The figure shows three views and two pictorial views of one solid part (mm, origin at its lowest corner). Answer the questions. A direction names the side the tool comes from. Coordinates: 2 decimals unless noted, no trailing zeros. Write each loop counter-clockwise with the first axis right and the second up, starting at its lowest first coordinate (ties: lowest second). Pieces come first, ordered by that corner, then holes. Notation, with made-up numbers: M 32.5,53.5 L 47.5,53.5 A14 cw 47.5,80.5 Z; hole C -14.5,58.25 d8. An arc over 180 degrees is marked long. Write item = value, one per line.
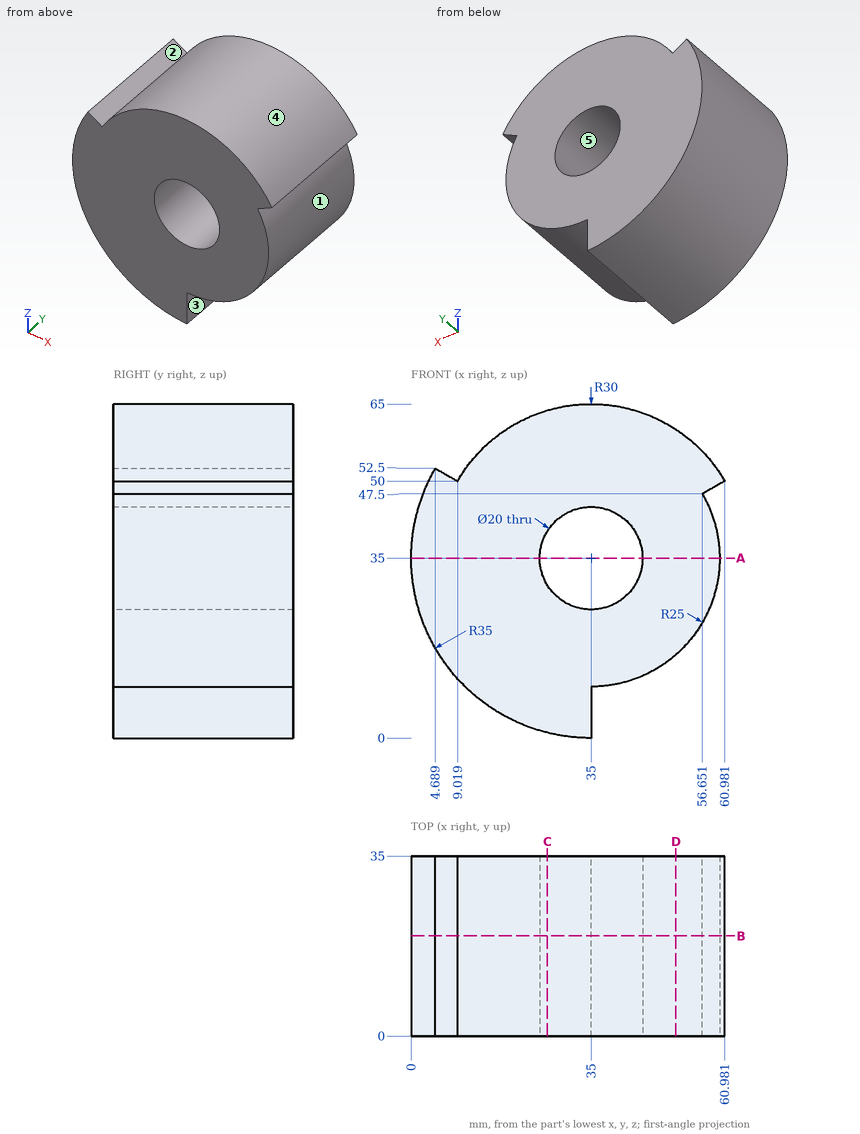
Item 1: Find section B-B (y = 19.5). Determine the outline of the cut face in (x, z).
Worked answers:
outline = M 4.69,52.5 A35 ccw 35,0 L 35,10 A25 ccw 56.65,47.5 L 60.98,50 A30 ccw 9.02,50 Z; hole C 35,35 d20
Item 2: Find section D-D (x = 51.5). Determine the outline of the cut face in (y, z) (1 decimal), and give its area (3 significant figures).
Worked answers:
outline = M 0,16.2 L 35,16.2 L 35,60.1 L 0,60.1 Z
area = 1,530 mm²
Item 3: Find section A-A (z = 35). Determine the outline of the cut face in (x, y).
Worked answers:
outline = M 0,0 L 25,0 L 25,35 L 0,35 Z; M 45,0 L 60,0 L 60,35 L 45,35 Z
Item 4: Which of the six approach directions +Z, -Z, +X, -X, +Y, -Y give full straight-line access (tool end or side, diameter ignored) to the marked faces 1 and 2?
Worked answers:
face_1 = +X, +Y, -Y
face_2 = +Z, +Y, -Y
Item 5: For a pull along Z with two mould halves and no side action, classify the marked faces 3, 4 and 5 as released by +Z, released by -Z, zero draft, split by the parting line, or undercut.
Worked answers:
face_3 = zero draft
face_4 = released by +Z
face_5 = undercut
Item 6: Flat-ended cylindrical pins translate along their axes: pin 1 (12 mm diameter, centred on y = 8, z = 57.5, fed in from +X) (1 decimal); pin 2 (1 mm diameter, centred on x = 25.5, y = 12.5, fed in from +Z); pin 3 (1 mm diameter, centred on y = 13, z = 45.5, fed in from +X). Find the tip coordinate at first contact, or state that the pin passes through.
Worked answers:
pin_1 = 60.1
pin_2 = 63.62
pin_3 = 57.91
Item 7: Consider line 1 along X through (y, z) = (16, 35); line 2 along Z through (x, y) = (30, 12); line 3 along Z through (x, y) = (43, 18) (1 decimal). Determine where each line is inside the solid, lowest interval first. Write a range as from..to.
Worked answers:
line_1 = 0..25, 45..60
line_2 = 0.36..26.34, 43.66..64.58
line_3 = 11.3..29, 41..63.9
Item 8: Find section C-C (x = 26.5). Determine the outline of the cut face in (y, z).
Worked answers:
outline = M 0,1.05 L 35,1.05 L 35,29.73 L 0,29.73 Z; M 0,40.27 L 35,40.27 L 35,63.77 L 0,63.77 Z
